Autodesk Inventor part; units mm, degrees
ref_plane "YZ Plane" through (0, 0, 0) normal (1, 0, 0) x (0, 1, 0)
ref_plane "XZ Plane" through (0, 0, 0) normal (0, 1, 0) x (-1, 0, 0)
ref_plane "XY Plane" through (0, 0, 0) normal (0, 0, 1) x (1, 0, 0)
sketch "Sketch1" plane through (0, 0, 0) normal (0, 0, 1) x (1, 0, 0)
  circle A0 centre (-295.4793, 52.101) radius 1.5875
  circle A1 centre (-281.943, 102.6189) radius 1.5875
  circle A2 centre (-259.8401, 150.0188) radius 1.5875
  circle A3 centre (-229.8421, 192.8604) radius 1.5875
  circle A4 centre (-219.9695, 210.9892) radius 1.5875
  circle A5 centre (-300.1694, 52.928) radius 1.5875
  circle A6 centre (-286.4183, 104.2477) radius 1.5875
  circle A7 centre (-263.9645, 152.4) radius 1.5875
  circle A8 centre (-233.4903, 195.9217) radius 1.5875
  circle A9 centre (-249.6775, 174.8261) radius 1.5875
  circle A10 centre (-276.2426, 128.814) radius 1.5875
  circle A11 centre (-294.4142, 78.888) radius 1.5875
  circle A12 centre (-303.6401, 26.5651) radius 1.5875
  circle A13 centre (-304.7338, 6.35) radius 1.5875
  circle A14 centre (-245.7763, 172.0944) radius 1.5875
  circle A15 centre (-271.9263, 126.8013) radius 1.5875
  circle A16 centre (-289.814, 77.6554) radius 1.5875
  circle A17 centre (-298.8958, 26.15) radius 1.5875
  arc A18 (-220.0163, 220.0163) -> (-311.15, 0) centre (0, 0) ccw
  line L0 (-311.15, 0) -> (0, 0)
  line L1 (0, 0) -> (-220.0163, 220.0163)
  arc A19 (-209.9135, 209.9135) -> (-296.8625, 0) centre (0, 0) ccw
  arc A20 (-220.0163, 220.0163) -> (-311.15, 0) centre (0, 0) ccw
  dimension "d0" = 593.725
extrude "Extrusion1" add sketch "Sketch1" along normal blind 6.35 contours L1 A19 L0 A18
sketch "Sketch2" plane through (0, 0, 6.35) normal (0, 0, 1) x (1, 0, 0)
  arc A0 (-220.0163, 220.0163) -> (-311.15, 0) centre (0, 0) ccw
  line L0 (-311.15, 0) -> (-296.8625, 0)
  line L1 (-311.15, 0) -> (-311.15, -6.35)
  line L2 (-311.15, -6.35) -> (-304.8, -6.35)
  line L3 (-304.8, -6.35) -> (-304.8, 0)
  dimension "d3" = 6.35
  dimension "d4" = 6.35
extrude "Extrusion2" add sketch "Sketch2" against normal blind 6.35
sketch "Sketch3" plane through (0, 0, 0) normal (0, 0, -1) x (-1, 0, 0)
  arc A0 (311.15, 0) -> (220.0163, 220.0163) centre (0, 0) ccw
  line L0 (311.15, -6.35) -> (311.15, 0)
  line L1 (220.0163, 220.0163) -> (177.0122, 220.0163)
  circle A1 centre (281.943, 102.6189) radius 1.5875
  circle A2 centre (263.9645, 152.4) radius 1.5875
  circle A3 centre (276.2426, 128.814) radius 1.5875
  circle A4 centre (245.7763, 172.0944) radius 1.5875
  circle A5 centre (249.6775, 174.8261) radius 1.5875
  circle A6 centre (286.4183, 104.2477) radius 1.5875
  circle A7 centre (295.4793, 52.101) radius 1.5875
  circle A8 centre (259.8401, 150.0188) radius 1.5875
  circle A9 centre (233.4903, 195.9217) radius 1.5875
  circle A10 centre (294.4142, 78.888) radius 1.5875
  circle A11 centre (289.814, 77.6554) radius 1.5875
  circle A12 centre (271.9263, 126.8013) radius 1.5875
  circle A13 centre (300.1694, 52.928) radius 1.5875
  circle A14 centre (219.9695, 210.9892) radius 1.5875
  circle A15 centre (229.8421, 192.8604) radius 1.5875
  arc A16 (311.15, 0) -> (224.8896, 215.0325) centre (0, 0) ccw
  line L2 (224.8896, 215.0325) -> (296.2163, 240.9933)
  line L3 (296.2163, 240.9933) -> (296.2163, 247.7508)
  line L4 (296.2163, 247.7508) -> (220.0163, 220.0163)
  line L5 (220.0163, 220.0163) -> (209.9135, 209.9135)
  arc A17 (293.5158, 44.45) -> (209.9135, 209.9135) centre (0, 0) ccw
  line L6 (293.5158, 44.45) -> (301.625, 44.45)
  line L7 (301.625, 44.45) -> (301.625, 0)
  line L8 (301.625, 0) -> (304.8, 0)
  line L9 (304.8, 0) -> (304.8, -6.35)
  line L10 (304.8, -6.35) -> (311.15, -6.35)
  line L11 (311.15, -6.35) -> (311.15, 0)
extrude "Extrusion3" add sketch "Sketch3" against normal blind 6.35 contours A0 L4 L3 L2
sketch "Sketch4" plane through (0, 0, 0) normal (0, 0, -1) x (-1, 0, 0)
  line L0 (209.9135, 209.9135) -> (220.0163, 220.0163)
  arc A0 (296.8625, 0) -> (209.9135, 209.9135) centre (0, 0) ccw
  arc A1 (311.15, 0) -> (224.8896, 215.0325) centre (0, 0) ccw
  line L1 (0, 0) -> (209.9135, 209.9135)
  line L2 (6.35, -6.35) -> (0, -6.35)
  line L3 (6.35, 0) -> (6.35, -6.35)
  line L4 (0, 0) -> (6.35, 0)
  line L5 (0, 0) -> (0, -6.35)
  line L6 (0, -6.35) -> (0, 0)
  line L7 (0, -6.35) -> (6.35, -6.35)
  line L8 (6.35, 0) -> (6.35, -6.35)
  line L9 (6.35, 0) -> (213.0645, 206.7145)
extrude "Extrusion4" add sketch "Sketch4" against normal blind 6.35
sketch "Sketch7" plane through (0, 0, 0) normal (0, 0, -1) x (-1, 0, 0)
  line L0 (220.0163, 220.0163) -> (0, 0)
  line L1 (296.2163, 247.7508) -> (220.0163, 220.0163)
  line L2 (0, 0) -> (220.0163, 220.0163)
  line L3 (202.0558, 206.5459) -> (211.036, 215.5261)
  line L4 (204.3008, 204.3008) -> (202.0558, 206.5459)
  line L5 (213.2811, 213.2811) -> (204.3008, 204.3008)
  line L6 (211.036, 215.5261) -> (213.2811, 213.2811)
  line L7 (-134.4395, 156.8901) -> (11.2253, 11.2253)
  line L8 (8.9803, 13.4704) -> (13.4704, 17.9605)
  line L9 (15.7154, 15.7154) -> (13.4704, 17.9605)
  line L10 (13.4704, 17.9605) -> (8.9803, 13.4704)
  line L11 (8.9803, 13.4704) -> (-8.9803, 31.4309)
  line L12 (15.7154, 15.7154) -> (24.6957, 24.6957)
  line L13 (24.6957, 24.6957) -> (22.4506, 26.9408)
  line L14 (22.4506, 26.9408) -> (202.0558, 206.5459)
  line L15 (202.0558, 206.5459) -> (204.3008, 204.3008)
  line L16 (204.3008, 204.3008) -> (213.2811, 213.2811)
  line L17 (213.2811, 213.2811) -> (211.036, 215.5261)
  line L18 (220.0163, 220.0163) -> (216.1966, 226.012)
  line L19 (211.036, 215.5261) -> (218.2689, 222.7591)
  line L20 (218.2689, 222.7591) -> (204.2902, 244.7013)
  line L21 (-8.9803, 31.4309) -> (204.2902, 244.7013)
  line L22 (204.3008, 204.3008) -> (202.0558, 206.5459)
  line L23 (211.036, 215.5261) -> (213.2811, 213.2811)
  line L24 (202.0558, 206.5459) -> (211.036, 215.5261)
  line L25 (213.2811, 213.2811) -> (204.3008, 204.3008)
  point P0 (8.9803, 8.9803)
  dimension "d19" = 25.4
  dimension "d20" = 102.5
extrude "Extrusion7" add sketch "Sketch7" against normal blind 6.35 contours L0 L4 L3 L6 | L19 L3 L14 L13 L0 L9 L8 L7 L21 L20 L18
sketch "Sketch8" plane through (0, 0, 0) normal (0, 0, -1) x (-1, 0, 0)
  line L0 (211.036, 215.5261) -> (218.2689, 222.7591)
  line L1 (218.2689, 222.7591) -> (204.2902, 244.7013)
  line L2 (296.2163, 247.7508) -> (220.0163, 220.0163)
  line L3 (238.4434, 230.102) -> (239.5293, 227.1184)
  line L4 (226.5093, 225.7583) -> (238.4434, 230.102)
  line L5 (227.5952, 222.7748) -> (226.5093, 225.7583)
  line L6 (239.5293, 227.1184) -> (227.5952, 222.7748)
  line L7 (220.5423, 223.5865) -> (221.6282, 220.603)
  line L8 (290.2492, 245.579) -> (278.3151, 241.2353)
  line L9 (289.1633, 248.5625) -> (290.2492, 245.579)
  line L10 (277.2292, 244.2188) -> (289.1633, 248.5625)
  line L11 (278.3151, 241.2353) -> (277.2292, 244.2188)
  line L12 (217.7712, 217.7712) -> (215.5261, 220.0163)
  line L13 (218.2689, 222.7591) -> (215.5261, 220.0163)
  line L14 (215.5261, 220.0163) -> (217.7712, 217.7712)
  line L15 (217.7712, 217.7712) -> (220.0163, 220.0163)
  line L16 (221.6282, 220.603) -> (220.0465, 220.0273)
  line L17 (221.6282, 220.603) -> (220.5423, 223.5865)
  line L18 (204.2902, 244.7013) -> (286.443, 274.6025)
  line L19 (295.1304, 250.7343) -> (296.2163, 247.7508)
  line L20 (295.1304, 250.7343) -> (286.443, 274.6025)
  line L21 (218.2689, 222.7591) -> (204.2902, 244.7013)
  line L22 (295.1304, 250.7343) -> (289.1633, 248.5625)
  line L23 (289.1633, 248.5625) -> (290.2492, 245.579)
  line L24 (290.2492, 245.579) -> (278.3151, 241.2353)
  line L25 (278.3151, 241.2353) -> (277.2292, 244.2188)
  line L26 (277.2292, 244.2188) -> (238.4434, 230.102)
  line L27 (238.4434, 230.102) -> (239.5293, 227.1184)
  line L28 (239.5293, 227.1184) -> (227.5952, 222.7748)
  line L29 (226.5093, 225.7583) -> (227.5952, 222.7748)
  line L30 (220.5423, 223.5865) -> (226.5093, 225.7583)
extrude "Extrusion8" add sketch "Sketch8" against normal blind 6.35 contours L0 L1 L18 L20 L22 L10 L26 L4 L30 L7 L2 L15 L12 | L9 L2 L11 L10 | L5 L4 L3 L2
sketch "Sketch11" plane through (0, 0, 0) normal (0, 0, -1) x (-1, 0, 0)
  line L0 (-8.9803, 31.4309) -> (8.9803, 13.4704)
  line L1 (296.2163, 240.9933) -> (296.2163, 247.7508)
  line L2 (204.3008, 204.3008) -> (24.6957, 24.6957)
  line L3 (-8.9803, 31.4309) -> (-33.676, 6.7352)
  line L4 (8.9803, 13.4704) -> (2.2451, 6.7352)
  line L5 (-33.676, 6.7352) -> (2.2451, 6.7352)
  dimension "d35" = 34.925
extrude "Extrusion11" add sketch "Sketch11" against normal blind 6.35
sketch "Sketch12" plane through (0, 0, 0) normal (0, 0, -1) x (-1, 0, 0)
  line L0 (204.2902, 244.7013) -> (-33.676, 6.7352)
  line L1 (204.3008, 204.3008) -> (24.6957, 24.6957)
  line L2 (-33.676, 6.7352) -> (-141.439, 114.4983)
  line L3 (-141.439, 114.4983) -> (-123.4785, 132.4588)
  line L4 (-123.4785, 132.4588) -> (-15.7154, 24.6957)
  line L5 (-134.7038, 112.2532) -> (-132.4588, 114.4983)
  line L6 (-132.4588, 114.4983) -> (-123.4785, 105.518)
  line L7 (-123.4785, 105.518) -> (-125.7236, 103.2729)
  line L8 (-125.7236, 103.2729) -> (-134.7038, 112.2532)
  line L9 (-60.6167, 42.6562) -> (-62.8618, 40.4112)
  line L10 (-62.8618, 40.4112) -> (-53.8815, 31.4309)
  line L11 (-53.8815, 31.4309) -> (-51.6365, 33.676)
  line L12 (-51.6365, 33.676) -> (-60.6167, 42.6562)
  dimension "d38" = 152.4
  dimension "d39" = 25.4
  dimension "d40" = 3.175
  dimension "d41" = 12.7
  dimension "d42" = 6.35
  dimension "d43" = 3.175
  dimension "d44" = 3.175
  dimension "d45" = 12.7
  dimension "d46" = 3.175
  dimension "d47" = 3.175
  dimension "d48" = 88.9
extrude "Extrusion12" add sketch "Sketch12" against normal blind 6.35
sketch "Sketch13" plane through (0, 0, 0) normal (0, 0, -1) x (-1, 0, 0)
  line L0 (224.8896, 215.0325) -> (296.2163, 240.9933)
  line L1 (296.2163, 240.9933) -> (296.2163, 247.7508)
  line L2 (296.2163, 247.7508) -> (290.2492, 245.579)
  line L3 (290.2492, 245.579) -> (289.1633, 248.5625)
  line L4 (289.1633, 248.5625) -> (295.1304, 250.7343)
  line L5 (295.1304, 250.7343) -> (286.443, 274.6025)
  line L6 (286.443, 274.6025) -> (204.2902, 244.7013)
  line L7 (278.3151, 241.2353) -> (239.5293, 227.1184)
  line L8 (238.4434, 230.102) -> (277.2292, 244.2188)
  line L9 (277.2292, 244.2188) -> (278.3151, 241.2353)
  line L10 (267.7713, 237.3977) -> (266.6854, 240.3812)
  line L11 (267.7713, 237.3977) -> (257.998, 264.2494)
  line L12 (267.7713, 237.3977) -> (269.9431, 231.4306)
extrude "Extrusion13" cut sketch "Sketch13" against normal blind 25.4 contours L12 L7 L9 L8 L11 L6 L5 L4 L3 L2 L1 L0
properties part number "Inner Rail" material "Polycarbonate, Clear"
Geometry check sheet. Reference: the model listing, model coordinates, mm. A direction names the side the tool comes from. Coordinates: 2 decimals unless noted, no trailing zeros. Order: outer loops, then holes, each group sorted by start corner. A loop starts at its lowest first (then second) coordinate and runs counter-clockwise, first axis right, second up.
Item 1: Tool access check on faces 1 (the flat face through (70.35, 79.33, 3.13)), 2 (the cylindrical face through (-275.714, 110.042, 3.131)), 3 (the flat face through (-252.762, 235.314, 3.131)). Record the directions out of +Z, -Z, +X, -X, +Y, -Y that give a thin tool (end or side, any length) a straight path to the whole face; none if there is none.
Item 2: Scan lines: line 1 along X through (y, z) = (179, 3); line 2 along X through (y, z) = (8, 6.25); line 3 along X through (y, z) = (96, 5.5). Record each from-to range of solid material in increasing order.
Item 3: Section check A-A (x = -142). Enter the section's corners in (y, z), plus the area to 3 significant figures.
Item 4: Depth check by flat-ended pin: pin 1 (1.9 mm diameter, centred on x = -219.97, y = 210.99, fed in from -Z); pin 2 (1 mm diameter, centred on x = -25, z = 5.5, fed in from +Y); pin 3 (1.5 mm diameter, centred on y = 143, z = 4.5, fed in from -X); pin 4 (3 mm diameter, centred on y = -2, z = 4.5, fed in from +X). Enter the tip coordinate at first touch or a pass-through.
Item 5: Mould release check, pull along X, two halves, no side actions. Record for faces 4 (the flat face through (86.8, 59.86, 3.13)), 5 (the flat face through (-253.85, 232.33, 3.13)), 6 (the flat face through (-262.4, 252.15, 3.13)), 7 (the flat face through (-108.26, 101.91, 3.13)): released by +X, released by -X, zero draft, split by the parting line, or undercut.
Item 6: Section check B-B (z = 5). Count the separate pieces of the cut face and the enclosed holes in it, plus the area to 3 significant figures.
Check sheet entries:
1. face 1: +Z, -Z, +Y
1. face 2: +Z, -Z, -Y
1. face 3: +Z, -Z
2. line 1: x = -254.51 to -236.83, -185.35 to -179, -174.51 to -138.59
2. line 2: x = -311.05 to -296.75, -14.35 to -8, -3.51 to 34.94
2. line 3: x = -295.97 to -280.91, -102.35 to -96, -91.51 to -55.59, 87.02 to 122.94
3. outline: (135.65, 0) - (142, 0) - (142, 6.35) - (135.65, 6.35) - close; (146.49, 0) - (182.41, 0) - (182.41, 6.35) - (146.49, 6.35) - close
3. area: 268 mm2
4. pin 1: passes through
4. pin 2: stops at y = 65.91
4. pin 3: stops at x = -276.73
4. pin 4: stops at x = 0
5. face 4: released by +X
5. face 5: undercut
5. face 6: released by -X
5. face 7: undercut
6. separate pieces: 1
6. enclosed holes: 23
6. area: 18,400 mm2
